Design review of the part built by this model. Coordinates are the model's own, in mm. Face numbers are marked on the shaded views. A direction names the side the tool comes from. Give positions to 0.01 mm unless a question says otherwise; leave off trailing zeros. Write each loop counter-clockwise with the first axis right and the second up, starting at its lowest first coordinate (ties: lowest second). Pieces come first, ordered by that corner, then holes. Notation, with made-up numbers: (7.5, 56.25) -> (39.5, 56.25) arc R20 cw to (39.5, 70.25) -> close; hole circle Ø1 at (-34, -33.5). An arc over 180 degrees is marked (long way). Write each question's results on one line, items separated by ' | '. Start each with the question number.
(1) Clearance check with flat-ended pins moving along their axes: pin 1 (5 mm diameter, centred on y = 330, z = 9.5, fed in from +X); pin 2 (5 mm diameter, centred on x = -194, z = -1, fed in from -Y); pin 3 (10 mm diameter, centred on y = 336, z = -7.5, fed in from -X). State where each tip first meets the part, or that it passes through.
(2) To check wall thickness, follow probe 1 along Y at (x, z) = (-249, 0.5); probe 2 along Y at (x, z) = (-436, 1.25); probe 3 along X at (y, z) = (515.5, 11). State the ranges of each line that lie inside material, in increasing order.
(3) Take a section at C-C (x = -450). State the section outline as (y, z) points.
(4) Take a section at A-A (z = 0). State the section outline as (x, y) points, plus the area to 3 significant figures.
(5) Take a section at B-B (y = 312). State the section outline as (x, z) points, plus the area to 3 significant figures.
(6) For the marked faces 1 and 2, list the 3-axis set-ups (+Z, -Z, +X, -X, +Y, -Y) from which the entire face can be reached by the end or side of a thin tool; tool diameter is ignored.
from build123d import *

# Parameters (mm, degrees)
SWEEP1_PROFILE_R    = 12.5
SKETCH2_R           = 12.5
BOSS_EXTRUDE4_DEPTH = 50.79
SKETCH11_R          = 12.5
CUT_EXTRUDE2_DEPTH  = 50.79


with BuildPart() as part:
    # Sweep1: sweep along a path in Sketch1
    with BuildLine(Plane.XY) as sweep1_path:
        Line((0, 0), (0, 495))
        ThreePointArc((0, 495), (-17.573593129, 537.426406871), (-60, 555))
        Line((-60, 555), (-480, 555))
    # Sweep1 profile (on start of the path) → Sweep1 (sweep)
    with BuildSketch(Plane.ZX):
        Circle(SWEEP1_PROFILE_R)
    sweep(path=sweep1_path.line)

    # Sketch2 → Boss-Extrude4 (add)
    with BuildSketch(Plane.XZ):
        Circle(SKETCH2_R)
    extrude(amount=BOSS_EXTRUDE4_DEPTH)

    # Sketch11 → Cut-Extrude2 (cut)
    with BuildSketch(Plane(origin=(0, 0, 0), x_dir=(0, 0, -1), z_dir=(1, 0, 0))):
        with Locations((0, 235)):
            Circle(SKETCH11_R)
    extrude(amount=CUT_EXTRUDE2_DEPTH, mode=Mode.SUBTRACT)


solid = part.part
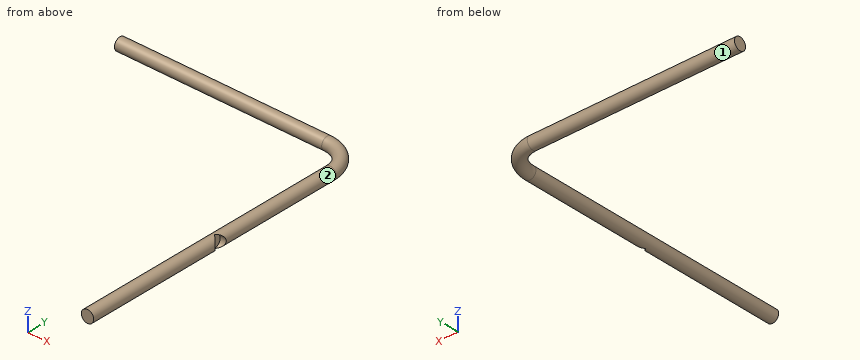
Report:
1) pin 1: x = 10.36 | pin 2: y = 542.5 | pin 3: x = -12.25
2) probe 1: 542.51 to 567.49 | probe 2: 542.56 to 567.44 | probe 3: -9.97 to 2.67
3) outline: circle Ø25 at (555, 0)
4) outline: (-480, 542.5) -> (-60, 542.5) arc R47.5 cw to (-12.5, 495) -> (-12.5, -50.79) -> (12.5, -50.79) -> (12.5, 222.5) -> (0, 222.5) -> (0, 247.5) -> (12.5, 247.5) -> (12.5, 495) arc R72.5 ccw to (-60, 567.5) -> (-480, 567.5) -> close | area: 26,200 mm2
5) outline: circle Ø25 at (0, 0) | area: 491 mm2
6) face 1: -X | face 2: -Y
